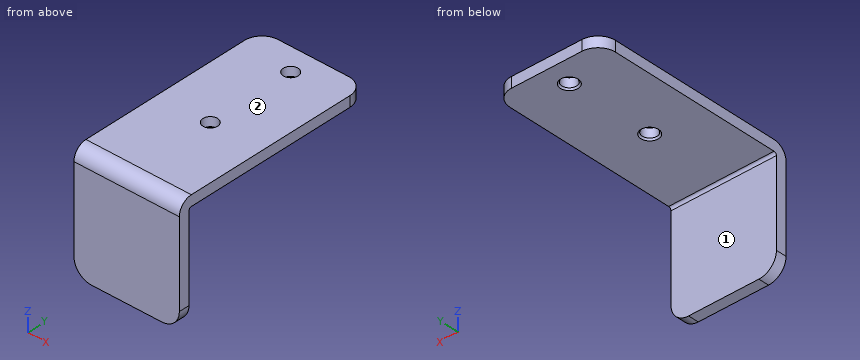
from build123d import *

# Parameters (mm, degrees)
BASE_FLANGE1_DEPTH          = 15
M5_TAPPED_HOLE1_D           = 4.2
M5_TAPPED_HOLE1_DEPTH       = 14
M5_TAPPED_HOLE1_CSINK_D     = 5.05
M5_TAPPED_HOLE1_CSINK_ANGLE = 90
M5_TAPPED_HOLE1_TIP         = 1.2618073
FILLET1_R                   = 5


# Sheet-metal steps are written as plain solids
with BuildPart() as part:
    # Sketch1 → Base-Flange1 (new, symmetric)
    with BuildSketch(Plane(origin=(0, 0, 0), x_dir=(0, 0, -1), z_dir=(1, 0, 0))):
        with BuildLine():
            Line((0, 0), (0, -54.2634))
            ThreePointArc((0, -54.2634), (0.215745145, -54.784254855), (0.7366, -55))
            Line((0.7366, -55), (30, -55))
            Line((30, -55), (30, -58))
            Line((30, -58), (0.7366, -58))
            ThreePointArc((0.7366, -58), (-1.905575199, -56.905575199), (-3, -54.2634))
            Line((-3, -54.2634), (-3, 0))
            Line((-3, 0), (0, 0))
        make_face()
    extrude(amount=BASE_FLANGE1_DEPTH, both=True)

    # M5 Tapped Hole1
    with Locations(Plane(origin=(0, 0, 0), x_dir=(-1, 0, 0), z_dir=(0, 0, -1))):
        with Locations((0, -32), (0, -7)):
            CounterSinkHole(M5_TAPPED_HOLE1_D / 2, M5_TAPPED_HOLE1_CSINK_D / 2, depth=M5_TAPPED_HOLE1_DEPTH, counter_sink_angle=M5_TAPPED_HOLE1_CSINK_ANGLE)
            with Locations((0, 0, -(M5_TAPPED_HOLE1_DEPTH + M5_TAPPED_HOLE1_TIP / 2))):  # 118° drill point
                Cone(0, M5_TAPPED_HOLE1_D / 2, M5_TAPPED_HOLE1_TIP, mode=Mode.SUBTRACT)

    # Fillet1
    fillet1_edges = [part.edges().sort_by_distance(p)[0] for p in [
        (15, 0, 1.5),
        (-15, 0, 1.5),
        (15, -56.5, -30),
        (-15, -56.5, -30),
    ]]
    fillet(fillet1_edges, radius=FILLET1_R)


solid = part.part
Could you check a few things on this model? Use its own coordinates, in mm. Face numbers are marked on the shaded views. A direction names the side the tool comes from. Coordinates: 2 decimals unless noted, no trailing zeros. Order: outer loops, then holes, each group sorted by start corner. A loop starts at its lowest first (then second) coordinate and runs counter-clockwise, first axis right, second up. Notation, with made-up numbers: (-9.5, -17.5) -> (41.5, -17.5) arc R31 ccw to (41.5, 20.5) -> close; hole circle Ø3 at (44, -32.5). An arc over 180 degrees is marked (long way). One line per item, written item: value. Start each with the question number.
1) Which directions (+Z, -Z, +X, -X, +Y, -Y) give clear straight access to the entire face, cutting with the end or side of a thin tool? Please do the marked faces 1 and 2.
2) Imagine slicing it at B-B on x = 0. List the corners of the cut face in (y, z) for me (3 decimals).
3) Imagine slicing it at D-D on y = -49. List the corners of the cut face in (x, z) for me, plus the area to 3 significant figures.
4) If I drill on L1, parallel to X at y = -7, z = 1; L2, parallel to Y at x = 0, z = 2.4; L3, parallel to Y at x = 0, z = 1.3, over which ranges is the centre line in solid material (lowest first)? Write a range as [from, to].
5) Imagine slicing it at C-C on x = 9.25. List the corners of the cut face in (y, z) for me.
6) Imagine slicing it at A-A on y = -32. List the corners of the cut face in (x, z) for me (3 decimals).
7) I'm going to push flat-ended pins straight in: pin 1 (10 mm diameter, centred on y = -8.5, z = -9.5, fed in from +X) (3 decimals); pin 2 (5.5 mm diameter, centred on x = 0, y = -7, fed in from -Z); pin 3 (8 mm diameter, centred on x = 10.5, z = -25.5, fed in from +Y); pin 4 (10 mm diameter, centred on y = -50.5, z = -19, fed in from -X). Where does each tip first touch, or does it pass through?
Answer list:
1. face 1: -Z, +X, -X, +Y
1. face 2: +Z, +X, -X, +Y, -Y
2. outline: (-58, -30) -> (-55, -30) -> (-55, -0.737) arc R0.737 cw to (-54.263, 0) -> (-34.525, 0) -> (-34.1, 0.425) -> (-34.1, 3) -> (-54.263, 3) arc R3.737 ccw to (-58, -0.737) -> close; (-29.9, 0.425) -> (-29.475, 0) -> (-9.525, 0) -> (-9.1, 0.425) -> (-9.1, 3) -> (-29.9, 3) -> close; (-4.9, 0.425) -> (-4.475, 0) -> (0, 0) -> (0, 3) -> (-4.9, 3) -> close
3. outline: (-15, 0) -> (15, 0) -> (15, 3) -> (-15, 3) -> close
3. area: 90.0 mm2
4. L1: x = [-15, -2.1], [2.1, 15]
4. L2: y = [-56.29, -34.1], [-29.9, -9.1], [-4.9, 0]
4. L3: y = [-57.4, -34.1], [-29.9, -9.1], [-4.9, 0]
5. outline: (-58, -30) -> (-55, -30) -> (-55, -0.74) arc R0.74 cw to (-54.26, 0) -> (0, 0) -> (0, 3) -> (-54.26, 3) arc R3.74 ccw to (-58, -0.74) -> close
6. outline: (-15, 0) -> (-2.525, 0) -> (-2.1, 0.425) -> (-2.1, 3) -> (-15, 3) -> close; (2.1, 0.425) -> (2.525, 0) -> (15, 0) -> (15, 3) -> (2.1, 3) -> close
7. pin 1: passes through
7. pin 2: stops at z = 0
7. pin 3: stops at y = -55
7. pin 4: stops at x = -15
